Design review of the part built by this model. Coordinates are the model's own, in mm. A direction names the side the tool comes from. Coordinates: 2 decimals unless noted, no trailing zeros. Loops run counter-clockwise (first coordinate to the right, second up) from the corner with the lowest first, then second, coordinate; pieces in that order, holes last. Notation, with made-up numbers: (85, 14.25) - (98, 14.25) arc R26 cw to (98, 36.25) - close; hole circle Ø4 at (11.25, 62). An arc over 180 degrees is marked (long way). One line per question, with ' | ' between items.
from build123d import *

# Parameters (mm, degrees)
SKETCH1_W             = 50
SKETCH1_H             = 44.8
BOSS_EXTRUDE1_DEPTH   = 4
CHAMFER1_SIZE         = 3
CHAMFER1_SIZE2        = 17.013845459
CHAMFER1_PART_2_SIZE  = 3
CHAMFER1_PART_2_SIZE2 = 17.013845459
CHAMFER1_PART_3_SIZE  = 3
CHAMFER1_PART_3_SIZE2 = 17.013845459
CHAMFER1_PART_4_SIZE  = 3
CHAMFER1_PART_4_SIZE2 = 17.013845459
SKETCH2_W             = 17
SKETCH2_H             = 11.8
SKETCH2_W_2           = 11
SKETCH2_H_2           = 5.8
CUT_EXTRUDE1_DEPTH    = 1
SKETCH3_W             = 10.2
SKETCH3_H             = 5.1
CUT_EXTRUDE2_DEPTH    = 3
SKETCH5_W             = 11
SKETCH5_H             = 5.8
BOSS_EXTRUDE2_DEPTH   = 1


with BuildPart() as part:
    # Sketch1 → Boss-Extrude1 (new body)
    with BuildSketch(Plane(origin=(0, 0, 0), x_dir=(1, 0, 0), z_dir=(0, 1, 0))):
        with Locations((25, -22.4)):
            Rectangle(SKETCH1_W, SKETCH1_H)
    extrude(amount=BOSS_EXTRUDE1_DEPTH)

    # Chamfer1
    chamfer1_edges = [part.edges().sort_by_distance(p)[0] for p in [
        (50, 4, 22.4),
    ]]
    chamfer1_side = [part.faces().sort_by_distance(p)[0] for p in [
        (50, 2, 22.4),
    ]]
    chamfer(chamfer1_edges, length=CHAMFER1_SIZE, length2=CHAMFER1_SIZE2, reference=chamfer1_side[0])

    # Chamfer1 part 2
    chamfer1_part_2_edges = [part.edges().sort_by_distance(p)[0] for p in [
        (25, 4, 0),
    ]]
    chamfer1_part_2_side = [part.faces().sort_by_distance(p)[0] for p in [
        (25, 2, 0),
    ]]
    chamfer(chamfer1_part_2_edges, length=CHAMFER1_PART_2_SIZE, length2=CHAMFER1_PART_2_SIZE2, reference=chamfer1_part_2_side[0])

    # Chamfer1 part 3
    chamfer1_part_3_edges = [part.edges().sort_by_distance(p)[0] for p in [
        (0, 4, 22.4),
    ]]
    chamfer1_part_3_side = [part.faces().sort_by_distance(p)[0] for p in [
        (0, 2, 22.4),
    ]]
    chamfer(chamfer1_part_3_edges, length=CHAMFER1_PART_3_SIZE, length2=CHAMFER1_PART_3_SIZE2, reference=chamfer1_part_3_side[0])

    # Chamfer1 part 4
    chamfer1_part_4_edges = [part.edges().sort_by_distance(p)[0] for p in [
        (25, 4, 44.8),
    ]]
    chamfer1_part_4_side = [part.faces().sort_by_distance(p)[0] for p in [
        (25, 2, 44.8),
    ]]
    chamfer(chamfer1_part_4_edges, length=CHAMFER1_PART_4_SIZE, length2=CHAMFER1_PART_4_SIZE2, reference=chamfer1_part_4_side[0])

    # Sketch2 → Cut-Extrude1 (cut)
    with BuildSketch(Plane(origin=(0, 4, 0), x_dir=(1, 0, 0), z_dir=(0, 1, 0))):
        with Locations((25, -22.4)):
            Rectangle(SKETCH2_W, SKETCH2_H)
        with Locations((25, -22.4)):
            Rectangle(SKETCH2_W_2, SKETCH2_H_2, mode=Mode.SUBTRACT)
    extrude(amount=-CUT_EXTRUDE1_DEPTH, mode=Mode.SUBTRACT)

    # Sketch3 → Cut-Extrude2 (cut)
    with BuildSketch(Plane(origin=(0, 4, 0), x_dir=(1, 0, 0), z_dir=(0, 1, 0))):
        with Locations((25, -22.45)):
            Rectangle(SKETCH3_W, SKETCH3_H)
    extrude(amount=-CUT_EXTRUDE2_DEPTH, mode=Mode.SUBTRACT)

    # Sketch5 → Boss-Extrude2 (add)
    with BuildSketch(Plane(origin=(0, 4, 0), x_dir=(1, 0, 0), z_dir=(0, 1, 0))):
        with Locations((25, -22.4)):
            Rectangle(SKETCH5_W, SKETCH5_H)
    extrude(amount=-BOSS_EXTRUDE2_DEPTH)


solid = part.part
Q1. To check wall thickness, follow line 1 along Y through (x, z) = (27.5, 21.5); line 2 along Y through (x, z) = (24, 14.5); line 3 along Y through (x, z) = (34.5, 31.5). State the ranges of each line that lie inside material, in increasing order.
Returned:
line 1: y = 0 to 1, 3 to 4 | line 2: y = 0 to 3.56 | line 3: y = 0 to 3.35
Q2. Take a section at C-C (y = 2.35). Give the boundary of the cut face in (x, z).
Returned:
outline: (7.66, 7.66) - (42.34, 7.66) - (42.34, 37.14) - (7.66, 37.14) - close; hole (19.9, 19.9) - (30.1, 19.9) - (30.1, 25) - (19.9, 25) - close
Q3. Take a section at A-A (x = 21.5). Give the boundary of the cut face in (y, z).
Returned:
outline: (0, 0) - (1, 0) - (3.91, 16.5) - (3, 16.5) - (3, 19.5) - (4, 19.5) - (4, 25.3) - (3, 25.3) - (3, 28.3) - (3.91, 28.3) - (1, 44.8) - (0, 44.8) - close; hole (1, 19.9) - (3, 19.9) - (3, 25) - (1, 25) - close
Q4. Take a section at B-B (z = 26.5). Give the boundary of the cut face in (x, y), plus the area to 3 significant figures.
Returned:
outline: (0, 0) - (50, 0) - (50, 1) - (33.5, 3.91) - (33.5, 3) - (16.5, 3) - (16.5, 3.91) - (0, 1) - close | area: 132 mm²
Q5. Draft analysis for pull direction X (two halves, no side actions). For faces 3 (the flat face through (25, 2, 19.9)), 4 (the flat face through (43.47, 2.15, 22.71)), 5 (the flat face through (6.53, 2.15, 22.71)), state which applies: +X half, -X half, draft (parallel to the pull), parting line (faces both ways), or undercut.
Returned:
face 3: undercut | face 4: +X half | face 5: -X half
Q6. For pin 1 (5 mm diameter, centred on x = 36.5, z = 12, fed in from +Y); pin 2 (8 mm diameter, centred on x = 26.5, z = 28, fed in from +Y); pin 3 (3 mm diameter, centred on x = 11.5, z = 10, fed in from +Y), all flat-tipped, find the tip position at first contact; note any pin that passes through.
Returned:
pin 1: stops at y = 3.53 | pin 2: stops at y = 4 | pin 3: stops at y = 3.03
Q7. Tool access review of faces 1 (the flat face through (25, 1, 22)), 2 (the flat face through (25, 0, 22)): name each direction out of +Z, -Z, +X, -X, +Y, -Y from which nothing blocks a thin tool from reaching the whole face with its end or side.
Returned:
face 1: none | face 2: +Z, -Z, +X, -X, -Y
Q8. Take a section at D-D (x = 37.5). Give the boundary of the cut face in (y, z), plus the area to 3 significant figures.
Returned:
outline: (0, 0) - (1, 0) - (3.2, 12.5) - (3.2, 32.3) - (1, 44.8) - (0, 44.8) - close | area: 116 mm²
